from build123d import *

# Parameters (mm, degrees)
F0_W        = 12.7
F0_H        = 33.7210557661
F1_DEPTH    = 7.62
F3_DEPTH    = 25.4
F4_T1_DEPTH = 59.8493549238
F4_T3_DEPTH = 38.8282991577
F5_T1_DEPTH = 27.94
F5_T3_DEPTH = 23.4635149399
F5_T5_DEPTH = 23.4635149399


# Not quite as in the source:
# - a fillet or chamfer that OpenCascade refuses, or shapes differently, is made with other operations: its cross-section is extruded or revolved along the edge and cut away or added


with BuildPart() as f1:
    # F0 (on Front) → F1 (new body)
    with BuildSketch(Plane.XZ):
        with Locations((-28.5366901662, 2.3533813655)):
            Rectangle(F0_W, F0_H)
    extrude(amount=F1_DEPTH)

    # F2 (on face) → F3 (cut)
    with BuildSketch(Plane.XZ.offset(7.62)):
        with BuildLine():
            ThreePointArc((-28.5366901662, -8.7627890215), (-30.9828768324, -11.2089756876), (-28.5366901662, -13.6551623538))
            Line((-28.5366901662, -13.6551623538), (-28.5366901662, -8.7627890215))
        make_face()
        with BuildLine():
            Line((-28.5366901662, -8.7627890215), (-28.5366901662, -13.6551623538))
            ThreePointArc((-28.5366901662, -13.6551623538), (-26.8069749865, -12.9386908673), (-26.0905035001, -11.2089756876))
            ThreePointArc((-26.0905035001, -11.2089756876), (-26.8069749865, -9.4792605079), (-28.5366901662, -8.7627890215))
        make_face()
    extrude(amount=-F3_DEPTH, mode=Mode.SUBTRACT)

    # F4: chamfer of 5.08 on 3 edges, made by hand

    # F4_s2 → F4_t1 (cut)
    with BuildSketch(Plane.XY.offset(-27.5712960964)):
        Polygon((-22.1866901662, -2.54), (-27.2666901662, -7.62), (-22.1866901662, -7.62), align=None)
        Polygon((-34.8866901662, -2.54), (-29.8066901662, -7.62), (-34.8866901662, -7.62), align=None)
    extrude(amount=F4_T1_DEPTH, mode=Mode.SUBTRACT)

    # F4_s4 → F4_t3 (cut)
    with BuildSketch(Plane.YZ.offset(-47.9508397451)):
        Polygon((-2.54, 19.2139092486), (-7.62, 14.1339092486), (-7.62, 19.2139092486), align=None)
    extrude(amount=F4_T3_DEPTH, mode=Mode.SUBTRACT)

    # F5: fillet of radius 5.08 on 6 edges, made by hand

    # F5_s2 → F5_t1 (cut)
    with BuildSketch(Plane.XZ.offset(-12.7)):
        with BuildLine():
            ThreePointArc((-29.8066901662, 19.2139092486), (-33.3987926146, 17.726011697), (-34.8866901662, 14.1339092486))
            Line((-34.8866901662, 14.1339092486), (-34.8866901662, 19.2139092486))
            Line((-34.8866901662, 19.2139092486), (-29.8066901662, 19.2139092486))
        make_face()
        with BuildLine():
            ThreePointArc((-27.2666901662, 19.2139092486), (-23.6745877178, 17.726011697), (-22.1866901662, 14.1339092486))
            Line((-22.1866901662, 14.1339092486), (-22.1866901662, 19.2139092486))
            Line((-22.1866901662, 19.2139092486), (-27.2666901662, 19.2139092486))
        make_face()
        with BuildLine():
            ThreePointArc((-22.1866901662, -9.4271465175), (-23.6745877178, -13.0192489659), (-27.2666901662, -14.5071465175))
            Line((-27.2666901662, -14.5071465175), (-22.1866901662, -14.5071465175))
            Line((-22.1866901662, -14.5071465175), (-22.1866901662, -9.4271465175))
        make_face()
        with BuildLine():
            ThreePointArc((-34.8866901662, -9.4271465175), (-33.3987926146, -13.0192489659), (-29.8066901662, -14.5071465175))
            Line((-29.8066901662, -14.5071465175), (-34.8866901662, -14.5071465175))
            Line((-34.8866901662, -14.5071465175), (-34.8866901662, -9.4271465175))
        make_face()
    extrude(amount=F5_T1_DEPTH, mode=Mode.SUBTRACT)

    # F5_s4 → F5_t3 (cut)
    with BuildSketch(Plane(origin=(-11.1509269725, -11.1509269725, -11.1509269725), x_dir=(-0.7071067812, 0.7071067812, 0), z_dir=(0.5773502692, 0.5773502692, 0.5773502692))):
        with BuildLine():
            ThreePointArc((16.4323078444, 27.2491898807), (14.5728987932, 25.3897808294), (13.8923078444, 22.8497808294))
            Line((13.8923078444, 22.8497808294), (13.8923078444, 25.7827201969))
            Line((13.8923078444, 25.7827201969), (16.4323078444, 27.2491898807))
        make_face()
    extrude(amount=F5_T3_DEPTH, mode=Mode.SUBTRACT)

    # F5_s6 → F5_t5 (cut)
    with BuildSketch(Plane(origin=(-7.8735331383, 7.8735331383, 7.8735331383), x_dir=(-0.7071067812, -0.7071067812, 0), z_dir=(-0.5773502692, 0.5773502692, 0.5773502692))):
        with BuildLine():
            ThreePointArc((23.9246664139, 3.949079929), (25.7840754651, 2.0896708777), (26.4646664139, -0.4503291223))
            Line((26.4646664139, -0.4503291223), (26.4646664139, 2.4826102452))
            Line((26.4646664139, 2.4826102452), (23.9246664139, 3.949079929))
        make_face()
    extrude(amount=F5_T5_DEPTH, mode=Mode.SUBTRACT)


solid = f1.part
The listing builds one solid part. Answer for the finished solid, in the listing's coordinates (mm). Round coordinates to 2 decimals unless told otherwise and drop trailing zeros. Loops run counter-clockwise (first coordinate to the right, second up) from the corner with the lowest first, then second, coordinate; pieces in that order, holes last. Notation, with made-up numbers: M 25.25,57 L 57.25,57 A32 ccw 57.25,88 Z; hole C 25,-29.5 d5. An arc over 180 degrees is marked long. Write each question's results on one line, items separated by ' | '. Start each with the question number.
1) Each of these flat-tipped pins is pushed along its axis until it touches: pin 1 (4 mm diameter, centred on y = -5.5, z = -4.5, fed in from -X); pin 2 (1 mm diameter, centred on x = -25.5, z = 14.5, fed in from -Y); pin 3 (5 mm diameter, centred on x = -32, z = -10.5, fed in from +Y). Where does it stop, or does it pass through?
2) Straight lines are drawn through the part: probe 1 along Z at (x, y) = (-30.75, -6); probe 2 along X at (y, z) = (-4, -12); probe 3 along Z at (x, y) = (-30.75, -4.5). For each, find the intervals that lie inside material, in ascending order.
3) Determine the mould class of faces 1 (the flat face through (-29, 0, 3)), 2 (the flat face through (-28.573, -3.593, 18.161)), 3 (the flat face through (-34.887, -1, 2)) for opening direction Y: pulls with the +Y half, pulls with the -Y half, needs draft (parallel to the pull), parting line crosses it, or undercut.
4) Find section A-A on z = -3. Write down the section's boundary in (x, y).
5) Find section B-B on z = -12. Write down the section's boundary in (x, y).
Final values:
1) pin 1: x = -33.93 | pin 2: y = -5.84 | pin 3: y = 0
2) probe 1: -14.42 to -12.25, -10.17 to 14.46 | probe 2: -33.43 to -30.85, -26.22 to -23.65 | probe 3: -14.42 to -12.25, -10.17 to 17.03
3) face 1: pulls with the +Y half | face 2: pulls with the -Y half | face 3: needs draft
4) outline: M -34.89,-2.54 L -29.81,-7.62 L -27.27,-7.62 L -22.19,-2.54 L -22.19,0 L -34.89,0 Z
5) outline: M -34.19,-3.24 L -30.85,-6.58 L -30.85,0 L -34.19,0 Z; M -26.22,-6.58 L -22.89,-3.24 L -22.89,0 L -26.22,0 Z
